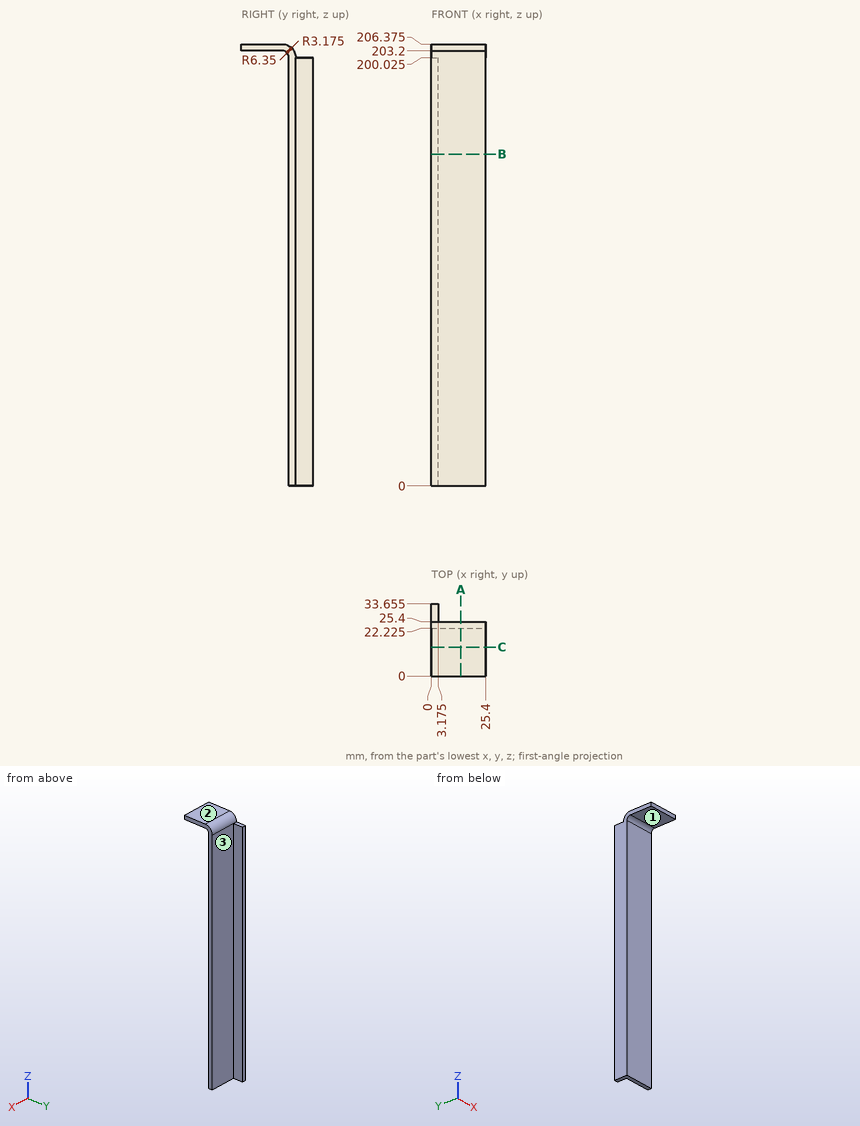
Verification items for this drawing (mm, ordinates from the low corner). A direction names the side the tool comes from. Coordinates: 2 decimals unless noted, no trailing zeros. Loops run counter-clockwise (first coordinate to the right, second up) from the corner with the lowest first, then second, coordinate; pieces in that order, holes last. Notation, with made-up numbers: (-38.5, 38.25) -> (-34.5, 38.25) arc R30 cw to (-34.5, 60.25) -> close; hole circle Ø4 at (-13, 33.5). An arc over 180 degrees is marked (long way). Answer in a Markdown table with one row per item. Add a question column.
1. Depth check by flat-ended pin: P1, Ø2, axis at y = 24, z = 123, coming from the -X side; P2, Ø2, axis at x = 13.5, z = 27, coming from the +Y side; P3, Ø4, axis at y = 28, z = 24.5, coming from the +X side (3 decimals); P4, Ø1.5, axis at x = 15, y = 14, coming from the -Z side. Enter the tip coordinate at first touch or a pass-through.
2. Section check B-B, the plane z = 155. Enter the section's corners in (x, y) (3 decimals).
3. Section check C-C, the plane y = 13.5. Enter the section's corners in (x, z) (3 decimals), then the cut area to 3 significant figures.
4. Section check A-A, the plane x = 13.75. Enter the section's corners in (y, z) (3 decimals).
5. Access from +Z, -Z, +X, -X, +Y, -Y to the whole of each face (thin tool, end or side, straight path). Record for the marked faces 1, 2 and 3.
6. Material ranges on probe 1 along Z at (x, y) = (14.5, 11.5) (3 decimals); probe 2 along Y at (x, z) = (11.5, 166) (3 decimals); probe 3 along X at (y, z) = (27.5, 167.5) (3 decimals), recorded low to high. Write a range as [from, to].
Derived:
| question | item | result |
|---|---|---|
| 1 | P1 | stops at x = 0 |
| 1 | P2 | stops at y = 25.4 |
| 1 | P3 | stops at x = 3.175 |
| 1 | P4 | stops at z = 203.2 |
| 2 | outline | (0, 22.225) -> (25.4, 22.225) -> (25.4, 25.4) -> (3.175, 25.4) -> (3.175, 33.655) -> (0, 33.655) -> close |
| 3 | outline | (0, 203.2) -> (25.4, 203.2) -> (25.4, 206.375) -> (0, 206.375) -> close |
| 3 | area | 80.6 mm² |
| 4 | outline | (0, 203.2) -> (19.05, 203.2) arc R3.175 cw to (22.225, 200.025) -> (22.225, 0) -> (25.4, 0) -> (25.4, 200.025) arc R6.35 ccw to (19.05, 206.375) -> (0, 206.375) -> close |
| 5 | face 1 | -Z, +X, -X, -Y |
| 5 | face 2 | +Z, +X, -X, +Y, -Y |
| 5 | face 3 | +Z, -Z, +X, +Y |
| 6 | probe 1 | z = [203.2, 206.375] |
| 6 | probe 2 | y = [22.225, 25.4] |
| 6 | probe 3 | x = [0, 3.175] |
